Model file for the job. Use its own axes, mm. Face numbers are marked on the shaded views. Coordinates: 2 decimals unless noted, no trailing zeros. Loops run counter-clockwise (first coordinate to the right, second up) from the corner with the lowest first, then second, coordinate; pieces in that order, holes last. Notation, with made-up numbers: M 22,30 L 29,30 A5 ccw 29,36 Z; hole C -5.75,43.5 d9. An arc over 180 degrees is marked long. One line per question, with ' | ' between items. Start each with the question number.
```python
from build123d import *

# Parameters (mm, degrees)
SKETCH_1_R      = 6
EXTRUDE_1_DEPTH = 10.4


with BuildPart() as part:
    # 草图1 → 凸台-拉伸1 (new, symmetric)
    with BuildSketch(Plane(origin=(0, 0, 0), x_dir=(1, 0, 0), z_dir=(0, 1, 0))):
        Polygon((4.330127019, 7.5), (-4.330127019, 7.5), (-8.660254038, 0), (-4.330127019, -7.5), (4.330127019, -7.5), (8.660254038, 0), align=None)
        with Locations(Location((0, 0, 0), (0, 0, 270))):
            Circle(SKETCH_1_R, mode=Mode.SUBTRACT)
    extrude(amount=EXTRUDE_1_DEPTH, both=True)

    # 草图3 → 切除-旋转1 (revolve, cut)
    with BuildSketch(Plane.XY, mode=Mode.PRIVATE) as cut_revolve_1_sk:
        Polygon((7.260254038, 10.4), (8.660254038, 8.4), (8.660254038, 10.4), align=None)
        Polygon((8.660254038, -10.4), (7.260254038, -10.4), (8.660254038, -8.4), align=None)
    revolve(cut_revolve_1_sk.sketch.rotate(Axis((0, 21.443940686, 0), (0, -1, 0)), 300.000000037), axis=Axis((0, 21.443940686, 0), (0, -1, 0)), mode=Mode.SUBTRACT)


solid = part.part
```
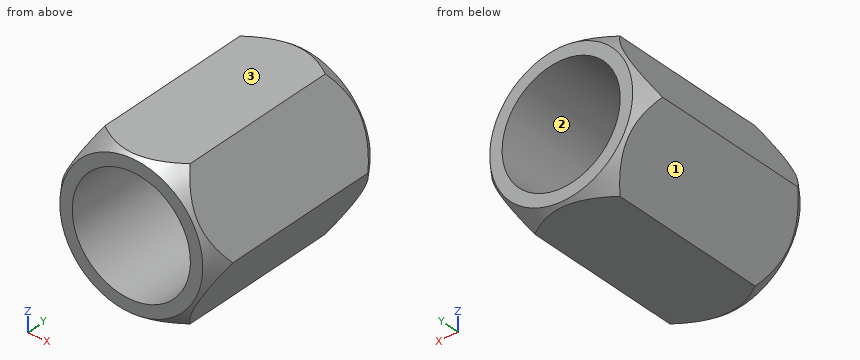
(1) Pin check, flat tips, straight feed: P1, Ø6, axis at x = 3, z = 4, coming from the -Y side; P2, Ø1, axis at x = 6, y = 2.5, coming from the -Z side; P3, Ø2, axis at y = 0, z = -2, coming from the -X side. Stop position of each tip, or through.
(2) Band-saw the part on B-B on y = -4.75. Write the cut outline in (x, z), then the cut area to 3 significant figures.
(3) Two-plate mould, pull along Z, no slides. Class the marked faces 1, 2 and 3: pulls with the +Z half, pulls with the -Z half, needs draft (parallel to the pull), parting line crosses it, or undercut.
(4) Band-saw the part on C-C on y = -9. Write the cut outline in (x, z).
(5) Drill centre lines: line 1 (Z direction, x = -0.25, y = 8); line 2 (X direction, y = -0.5, z = -3.25); line 3 (Z direction, x = -3, y = -2.5). Where is each one in solid material? Low to high. Write a range as [from, to].
(6) Band-saw the part on A-A on x = 0. Write the cut outline in (y, z).
Computed values:
1) P1: y = -10.4 | P2: z = -5.47 | P3: x = -8.08
2) outline: M -8.66,0 L -4.33,-7.5 L 4.33,-7.5 L 8.66,0 L 4.33,7.5 L -4.33,7.5 Z; hole C 0,0 d12 | area: 81.8 mm^2
3) face 1: pulls with the -Z half | face 2: undercut | face 3: pulls with the +Z half
4) outline: M -8.2,-0.79 L -4.79,-6.71 A8.24 ccw -3.41,-7.5 L 3.41,-7.5 A8.24 ccw 4.79,-6.71 L 8.2,-0.79 A8.24 ccw 8.2,0.79 L 4.79,6.71 A8.24 ccw 3.41,7.5 L -3.41,7.5 A8.24 ccw -4.79,6.71 L -8.2,0.79 A8.24 ccw Z; hole C 0,0 d12
5) line 1: [-7.5, -5.99], [5.99, 7.5] | line 2: [-6.78, -5.04], [5.04, 6.78] | line 3: [-7.5, -5.2], [5.2, 7.5]
6) outline: M -10.4,-7.26 L -10.06,-7.5 L 10.06,-7.5 L 10.4,-7.26 L 10.4,-6 L -10.4,-6 Z; M -10.4,6 L 10.4,6 L 10.4,7.26 L 10.06,7.5 L -10.06,7.5 L -10.4,7.26 Z
